Autodesk Inventor part; units mm, degrees
ref_plane "YZ Plane" through (0, 0, 0) normal (1, 0, 0) x (0, 1, 0)
ref_plane "XZ Plane" through (0, 0, 0) normal (0, 1, 0) x (-1, 0, 0)
ref_plane "XY Plane" through (0, 0, 0) normal (0, 0, 1) x (1, 0, 0)
sketch "草图1" plane through (0, 0, 0) normal (0, 0, 1) x (1, 0, 0)
  line L0 (-16.8, 24.9) -> (-16.8, 21.24)
  line L1 (-16.8, 21.24) -> (-21.2406, 16.7994)
  line L2 (-21.2406, 16.7994) -> (-24.9006, 16.7994)
  line L3 (16.8, -24.9) -> (16.8, -21.24)
  line L4 (16.8, -21.24) -> (21.2406, -16.7994)
  line L5 (21.2406, -16.7994) -> (24.9006, -16.7994)
  line L6 (-24.9006, 16.7994) -> (16.8, -24.9)
  line L7 (0, 0) -> (-0.1347, -0.1347)
  line L8 (22.4746, -22.7439) -> (22.4746, -22.7439)
  line L9 (-15, 15) -> (-15, 23.1001)
  line L10 (15, -15) -> (23.1012, -15)
  line L11 (-15, 23.1001) -> (-16.8, 24.9)
  line L12 (23.1012, -15) -> (24.9006, -16.7994)
  line L13 (-15, 15) -> (15, -15)
extrude "拉伸1" add sketch "草图1" along normal blind 15 and the other way blind 15
sketch "草图2" plane through (-15, 15, -15) normal (0.7071068, 0.7071068, 0) x (-0.7071068, 0.7071068, 0)
  point P0 (-21.2132, 15)
  point P1 (-21.2132, 15)
hole "孔1" at (0, 0, 0) direction (-0.7071068, -0.7071068, 0) diameter 23 end through all counterbore diameter 25.4 counterbore depth 1.1
sketch "草图3" plane through (-15, 15, -15) normal (0.7071068, 0.7071068, 0) x (-0.7071068, 0.7071068, 0)
  point P0 (-21.2132, 15)
sketch "草图4" plane through (-15, 15, -15) normal (0.7071068, 0.7071068, 0) x (-0.7071068, 0.7071068, 0)
  point P0 (-21.2132, 15)
sketch "草图5" plane through (-15, 15, -15) normal (0.7071068, 0.7071068, 0) x (-0.7071068, 0.7071068, 0)
  circle A0 centre (-21.2132, 15) radius 12.7
  circle A1 centre (-21.2132, 15) radius 13.2
  dimension "d18" = 0.5
  dimension "d19" = 25.4
extrude "拉伸2" add sketch "草图5" along normal blind 1.5 contours A0 | A1
sketch "草图6" plane through (1.0607, 1.0607, 0) normal (0.7071068, 0.7071068, 0) x (-0.7071068, 0.7071068, 0)
  point P0 (0, 0)
  point P1 (0, 0)
hole "孔2" at (1.0607, 1.0607, 0) direction (-0.7071068, -0.7071068, 0) diameter 25.4 end up to surface
fillet "圆角1" radius 0.5 1 edges at (-16.8, 24.9, 0)
fillet "圆角2" radius 0.5 1 edges at (-24.9006, 16.7994, 0)
fillet "圆角3" radius 0.5 1 edges at (24.9006, -16.7994, 0)
fillet "圆角4" radius 0.5 1 edges at (16.8, -24.9, 0)
sketch "草图7" plane through (-15, 15, -15) normal (0.7071068, 0.7071068, 0) x (-0.7071068, 0.7071068, 0)
  point P0 (-21.2132, 15)
equation "\"d15\" = Thickness"
equation "\"BendRadius\" = Thickness"
equation "\"BendReliefWidth\" = Thickness"
equation "\"BendReliefDepth\" = 0.5 * Thickness"
equation "\"CornerReliefSize\" = 4 * Thickness"
equation "\"MinimumRemnant\" = 2 * Thickness"
equation "\"TransitionRadius\" = BendRadius"
equation "\"JacobiRadiusSize\" = BendRadius"
equation "\"GapSize\" = Thickness"
properties part number "fenguangjing"
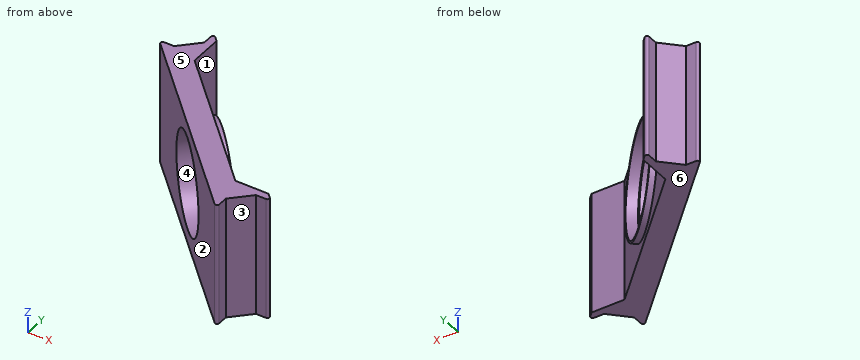
Source: CAD feature listing. Evaluate the final solid. Frame: model axes, mm. Face numbers are marked on the shaded views. A direction names the side the tool comes from. Give positions to 0.01 mm unless a question says otherwise; leave off trailing zeros. Write each loop counter-clockwise with the first axis right and the second up, starting at its lowest first coordinate (ties: lowest second). Pieces come first, ordered by that corner, then holes. Notation, with made-up numbers: M 77.25,-25.5 L 132.25,-25.5 A8 ccw 132.25,-11.5 Z; hole C 50,69 d4. An arc over 180 degrees is marked long. Return JSON: item names as keys, results as strings. Group by question number.
1) First-contact query: pin 1 Ø4 at (x, z) = (-17.5, -1.5) entering from -Y; pin 2 Ø2.5 at (x, z) = (22, -2.5) entering from -Y; pin 3 Ø4 at (x, z) = (-11.5, 10) entering from -Y. Flat tips, straight axial feed; report the tip coordinate or a pass-through.
2) Cut plane D-D, the plane y = 19. Output: boundary loops of the cut face in (x, z).
3) Cut plane C-C, the plane z = 5.75. Output: boundary loops of the cut face in (x, y), then the cut area to 3 significant figures.
4) Set-up query: the marked faces 1 and 2. Return all of +Z, -Z, +X, -X, +Y, -Y with unobstructed straight access to the full face (end or side cutting, diameter ignored); none if empty.
5) Ray query, L1, parallel to X at y = 22.5, z = -4.5; L2, parallel to X at y = -14.5, z = 3; L3, parallel to Y at x = -14, z = -3.25. Return the intervals inside material, ascending.
6) Cut plane A-A, the plane z = 2.75. Output: boundary loops of the cut face in (x, y).
7) Cut plane B-B, the plane x = 19.5. Output: boundary loops of the cut face in (y, z).
8) Draft query along Z for the marked faces 3, 4, 5 and 6. Return one class per face: released by +Z, released by -Z, zero draft, split by the parting line, or undercut.
Data:
{
 "1": {"pin 1": "stops at y = 7.4", "pin 2": "stops at y = -17.29", "pin 3": "stops at y = 1.4"},
 "2": {"outline": "M -19.04,-15 L -15,-15 L -15,15 L -19.04,15 Z"},
 "3": {"outline": "M -24.05,15.95 L -11.09,2.99 L -7.82,6.26 L -8.78,7.23 L -6.95,9.07 L -7.34,9.46 L -8.4,8.4 L -15,15 L -15,23.1 L -15.95,24.05 A0.5 ccw -16.8,23.69 L -16.8,21.24 L -21.24,16.8 L -23.69,16.8 A0.5 ccw Z; M 2.99,-11.09 L 15.95,-24.05 A0.5 ccw 16.8,-23.69 L 16.8,-21.24 L 21.24,-16.8 L 23.69,-16.8 A0.5 ccw 24.05,-15.95 L 23.1,-15 L 15,-15 L 8.4,-8.4 L 9.46,-7.34 L 9.07,-6.95 L 7.23,-8.78 L 6.26,-7.82 Z", "area": "237 mm²"},
 "4": {"face 1": "+Z, -Z, +X, +Y", "face 2": "+Z, -Z, -X, -Y"},
 "5": {"L1": "x = -16.8 to -15", "L2": "x = 6.4 to 14.5", "L3": "y = 5.9 to 14"},
 "6": {"outline": "M -24.05,15.95 L -11.95,3.85 L -8.67,7.12 L -9.55,7.99 L -7.71,9.83 L -8.07,10.19 L -9.13,9.13 L -15,15 L -15,23.1 L -15.95,24.05 A0.5 ccw -16.8,23.69 L -16.8,21.24 L -21.24,16.8 L -23.69,16.8 A0.5 ccw Z; M 3.85,-11.95 L 15.95,-24.05 A0.5 ccw 16.8,-23.69 L 16.8,-21.24 L 21.24,-16.8 L 23.69,-16.8 A0.5 ccw 24.05,-15.95 L 23.1,-15 L 15,-15 L 9.13,-9.13 L 10.19,-8.07 L 9.83,-7.71 L 7.99,-9.55 L 7.12,-8.67 Z"},
 "7": {"outline": "M -18.54,-15 L -15,-15 L -15,15 L -18.54,15 Z"},
 "8": {"face 3": "zero draft", "face 4": "undercut", "face 5": "released by +Z", "face 6": "released by -Z"}
}
